```python
from build123d import *

# Parameters (mm, degrees)
SKETCH1_W           = 60
SKETCH1_H           = 120
SKETCH1_R           = 3.25
BOSS_EXTRUDE1_DEPTH = 3
CHAMFER1_SIZE       = 3


with BuildPart() as part:
    # Sketch1 → Boss-Extrude1 (new body)
    with BuildSketch(Plane.XY):
        with Locations((12.372881356, -8.156527448)):
            Rectangle(SKETCH1_W, SKETCH1_H)
        with Locations((-4.281987853, 36.843472552)):
            Circle(SKETCH1_R, mode=Mode.SUBTRACT)
        with Locations((25.718012147, 36.843472552)):
            Circle(SKETCH1_R, mode=Mode.SUBTRACT)
        with Locations((-4.281987853, 6.843472552)):
            Circle(SKETCH1_R, mode=Mode.SUBTRACT)
        with Locations((25.718012147, 6.843472552)):
            Circle(SKETCH1_R, mode=Mode.SUBTRACT)
        with Locations((-4.281987853, -23.156527448)):
            Circle(SKETCH1_R, mode=Mode.SUBTRACT)
        with Locations((25.718012147, -23.156527448)):
            Circle(SKETCH1_R, mode=Mode.SUBTRACT)
        with Locations((-4.281987853, -53.156527448)):
            Circle(SKETCH1_R, mode=Mode.SUBTRACT)
        with Locations((25.718012147, -53.156527448)):
            Circle(SKETCH1_R, mode=Mode.SUBTRACT)
    extrude(amount=BOSS_EXTRUDE1_DEPTH)

    # Chamfer1
    chamfer1_edges = [part.edges().sort_by_distance(p)[0] for p in [
        (-17.627118644, 51.843472552, 1.5),
        (42.372881356, 51.843472552, 1.5),
        (42.372881356, -68.156527448, 1.5),
        (-17.627118644, -68.156527448, 1.5),
    ]]
    chamfer(chamfer1_edges, length=CHAMFER1_SIZE)


solid = part.part
```
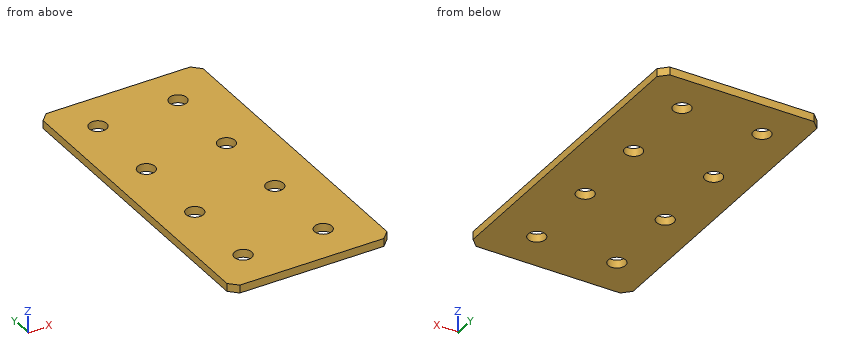
CAD build for the part. Positions are in the model's coordinates, mm. Give positions to 0.01 mm unless a question says otherwise; leave off trailing zeros. Loops run counter-clockwise (first coordinate to the right, second up) from the corner with the lowest first, then second, coordinate; pieces in that order, holes last. Notation, with made-up numbers: (-1, -30) - (40, -30) arc R14 ccw to (40, -21) - close; hole circle Ø9 at (-12.75, -14.75). An arc over 180 degrees is marked (long way). Put each result on its own line as item: value.
Q1. Probe line 1 along X through (y, z) = (-24.5, 0.8); line 2 along Y through (x, z) = (-6, 1.6); line 3 along Y through (x, z) = (23, 1.85). List the from-to ranges inside material, lowest first.
Filled in:
line 1: x = -17.63 to -7.24, -1.32 to 22.76, 28.68 to 42.37
line 2: y = -68.16 to -55.92, -50.4 to -25.92, -20.4 to 4.08, 9.6 to 34.08, 39.6 to 51.84
line 3: y = -68.16 to -54.94, -51.37 to -24.94, -21.37 to 5.06, 8.63 to 35.06, 38.63 to 51.84
Q2. Flat gauge pin, fed straight in: pin 1 (1.5 mm diameter, centred on x = 29.5, y = -4, fed in from -Z). Where does the tip first touch, or does it go through?
Filled in:
pin 1: stops at z = 0
Q3. Slice it at A-A (y = -51.5). Give the cut face in (x, z), plus the area to 3 significant figures.
Filled in:
outline: (-17.63, 0) - (-7.08, 0) - (-7.08, 3) - (-17.63, 3) - close; (-1.49, 0) - (22.92, 0) - (22.92, 3) - (-1.49, 3) - close; (28.51, 0) - (42.37, 0) - (42.37, 3) - (28.51, 3) - close
area: 146 mm²
Q4. Slice it at B-B (z = 2). Give the number of separate pieces and of enclosed holes in the cut face, plus the area to 3 significant figures.
Filled in:
separate pieces: 1
enclosed holes: 8
area: 6,920 mm²
